For this review, take the finished solid that the model builds, in its own axes (mm). A direction names the side the tool comes from. Give positions to 0.01 mm unless a question says otherwise; leave off trailing zeros. Order: outer loops, then holes, each group sorted by start corner. A loop starts at its lowest first (then second) coordinate and runs counter-clockwise, first axis right, second up. Notation, with made-up numbers: (-40, 66) - (0, 66) arc R29 ccw to (0, 101) - close; hole circle Ø11 at (0.25, 20.5). An arc over 180 degrees is marked (long way). One line per item, written item: value.
```python
from build123d import *

# Parameters (mm, degrees)
F1_DEPTH = 2.286
F2_D     = 1.778


with BuildPart() as f1:
    # F0 (on Front) → F1 (new body)
    with BuildSketch(Plane.XZ):
        with BuildLine():
            ThreePointArc((-44.9743270874, 48.1504499912), (-47.139991973, 50.3428364156), (-49.3587702513, 48.2042187354))
            Line((-49.3587702513, 48.2042187354), (-49.3587702513, 32.7516756952))
            ThreePointArc((-49.3587702513, 32.7516756952), (-47.1665486693, 30.5594541132), (-44.9743270874, 32.7516756952))
            Line((-44.9743270874, 32.7516756952), (-44.9743270874, 48.1504499912))
        make_face()
        with BuildLine():
            ThreePointArc((-48.060906813, 48.1504499912), (-47.1693925898, 49.0419642144), (-46.2778783666, 48.1504499912))
            Line((-46.2778783666, 48.1504499912), (-46.2778783666, 32.7516756952))
            ThreePointArc((-46.2778783666, 32.7516756952), (-47.1693925898, 31.860161472), (-48.060906813, 32.7516756952))
            Line((-48.060906813, 32.7516756952), (-48.060906813, 48.1504499912))
        make_face(mode=Mode.SUBTRACT)
    extrude(amount=F1_DEPTH)

    # F2 (through all)
    with Locations(Plane(origin=(0, 0, 0), x_dir=(1, 0, 0), z_dir=(0, 1, 0))):
        with Locations((-47.1668783666, -48.1504499912), (-47.1665486693, -32.7516756952)):
            Hole(F2_D / 2)


solid = f1.part
```
(1) Take a section at C-C (x = -47.05). Write out the cut boundary in (y, z), then the cut area to 3 significant figures.
Answers below:
outline: (-2.29, 30.56) - (0, 30.56) - (0, 31.87) - (-2.29, 31.87) - close; (-2.29, 49.03) - (0, 49.03) - (0, 50.34) - (-2.29, 50.34) - close
area: 5.97 mm^2
(2) Take a section at D-D (x = -45.25). Write out the cut boundary in (y, z).
Answers below:
outline: (-2.29, 31.69) - (0, 31.69) - (0, 49.21) - (-2.29, 49.21) - close
(3) Draft analysis for pull direction X (two halves, no side actions). For faces 1 (the face through (-47.21, -1.13, 30.56)), 2 (the face through (-48.061, -1, 40)), 3 (the face through (-46, 0, 41)), state which applies: pulls with the +X half, pulls with the -X half, needs draft (parallel to the pull), parting line crosses it, or undercut.
Answers below:
face 1: parting line crosses it
face 2: undercut
face 3: needs draft
(4) Machinability: for faces 4 (the face through (-47.19, -1.13, 49.04)), 5 (the face through (-44.974, -1, 40)), which of the approach directions +Z, -Z, +X, -X, +Y, -Y give a long, thin tool a straight path to every point of the face, cutting with its end or side? Answer none if there is none.
Answers below:
face 4: +Y, -Y
face 5: +Z, -Z, +X, +Y, -Y
(5) Wall thickness on line 1 (X direction, y = -0.75, z = 45.75); line 2 (Z direction, x = -46.7, y = -1.4); line 3 (Z direction, x = -46.85, y = -0.5): over which ranges is each line inside the solid? List them lowest first. Write a range as from..to.
Answers below:
line 1: x = -49.36..-48.06, -46.28..-44.97
line 2: z = 30.61..31.99, 48.91..50.29
line 3: z = 30.58..31.92, 48.98..50.32
(6) Take a section at A-A (z = 36.25). Write out the cut boundary in (x, y), then the cut area to 3 significant figures.
Answers below:
outline: (-49.36, -2.29) - (-48.06, -2.29) - (-48.06, 0) - (-49.36, 0) - close; (-46.28, -2.29) - (-44.97, -2.29) - (-44.97, 0) - (-46.28, 0) - close
area: 5.95 mm^2
(7) Take a section at B-B (y = -0.3). Write out the cut boundary in (x, z), then the cut area to 3 significant figures.
Answers below:
outline: (-49.36, 32.75) arc R2.19 ccw to (-44.97, 32.75) - (-44.97, 48.15) arc R2.19 ccw to (-49.36, 48.2) - close; hole (-48.06, 32.75) arc R0.89 ccw to (-46.38, 32.34) arc R0.89 ccw to (-46.28, 32.78) - (-46.28, 48.15) arc R0.89 ccw to (-48.06, 48.15) - close
area: 52.7 mm^2
